from build123d import *

# Parameters (mm, degrees)
SKETCH2_W           = 101.6
SKETCH2_H           = 88.9
BOSS_EXTRUDE1_DEPTH = 3.175
SKETCH3_R           = 1.4605
CUT_EXTRUDE1_DEPTH  = 68.576054376
SKETCH5_W           = 3.175
SKETCH5_H           = 16.51
CUT_EXTRUDE2_DEPTH  = 68.576054376


with BuildPart() as part:
    # Sketch2 → Boss-Extrude1 (new body)
    with BuildSketch(Plane(origin=(0, 0, 0), x_dir=(1, 0, 0), z_dir=(0, 1, 0))):
        Rectangle(SKETCH2_W, SKETCH2_H)
    extrude(amount=BOSS_EXTRUDE1_DEPTH)

    # Sketch3 → Cut-Extrude1 (cut, through all)
    with BuildSketch(Plane(origin=(0, 3.175, 0), x_dir=(1, 0, 0), z_dir=(0, 1, 0))):
        with Locations(Location((-25.4, 0, 0), (0, 0, 270))):
            Circle(SKETCH3_R)
        with Locations(Location((25.4, 0, 0), (0, 0, 270))):
            Circle(SKETCH3_R)
    extrude(amount=-CUT_EXTRUDE1_DEPTH, mode=Mode.SUBTRACT)

    # Sketch5 → Cut-Extrude2 (cut, through all)
    with BuildSketch(Plane(origin=(0, 3.175, 0), x_dir=(1, 0, 0), z_dir=(0, 1, 0))):
        with Locations((-3.175, -1.713817512)):
            Rectangle(SKETCH5_W, SKETCH5_H)
        with Locations((3.175, -1.713817512)):
            Rectangle(SKETCH5_W, SKETCH5_H)
    extrude(amount=-CUT_EXTRUDE2_DEPTH, mode=Mode.SUBTRACT)


solid = part.part
Can you work these out from the model? Positions are in its coordinate system, mm. A direction names the side the tool comes from. Give positions to 0.01 mm unless a question says otherwise; leave off trailing zeros. Loops run counter-clockwise (first coordinate to the right, second up) from the corner with the lowest first, then second, coordinate; pieces in that order, holes last. Notation, with made-up numbers: (-16, -29.5) -> (42, -29.5) arc R29 ccw to (42, -2.5) -> close; hole circle Ø10 at (32.25, -5). An arc over 180 degrees is marked (long way). Return JSON: item names as keys, results as strings.
Q1. I want a section at B-B, the plane z = 0. List the corners of the cut face in (x, y) for me (1 decimal).
Checks:
{"outline": "(-50.8, 0) -> (-26.9, 0) -> (-26.9, 3.2) -> (-50.8, 3.2) -> close; (-23.9, 0) -> (-4.8, 0) -> (-4.8, 3.2) -> (-23.9, 3.2) -> close; (-1.6, 0) -> (1.6, 0) -> (1.6, 3.2) -> (-1.6, 3.2) -> close; (4.8, 0) -> (23.9, 0) -> (23.9, 3.2) -> (4.8, 3.2) -> close; (26.9, 0) -> (50.8, 0) -> (50.8, 3.2) -> (26.9, 3.2) -> close"}
Q2. We'd pull the mould along Z, two halves only. Please class faces 3 (the face through (3, 2, -6.541)), 4 (the face through (-1, 2, 44.45)), 5 (the face through (50.8, 2, 1)): released by +Z, released by -Z, zero draft, split by the parting line, or undercut.
Checks:
{"face 3": "undercut", "face 4": "released by +Z", "face 5": "zero draft"}
Q3. I need wall thicknesses on probe 1 along X at (y, z) = (1.7, 0); probe 2 along X at (y, z) = (1.4, 4.5); probe 3 along X at (y, z) = (1.45, 0.5). Which ranges of each line are inside material? Lowest first, please.
Checks:
{"probe 1": "x = -50.8 to -26.86, -23.94 to -4.76, -1.59 to 1.59, 4.76 to 23.94, 26.86 to 50.8", "probe 2": "x = -50.8 to -4.76, -1.59 to 1.59, 4.76 to 50.8", "probe 3": "x = -50.8 to -26.77, -24.03 to -4.76, -1.59 to 1.59, 4.76 to 24.03, 26.77 to 50.8"}
Q4. For pin 1 Ø1.8 at (x, z) = (25.4, 0) entering from -Y, with a flat end and sliding along its axis, tell me the tip position at first contact or that it passes through.
Checks:
{"pin 1": "passes through"}
Q5. On a 3-axis mill with a long thin cutter (end or side, diameter ignored), from which of +Z, -Z, +X, -X, +Y, -Y can I reach the whole of each face in a straight line? I mean faces 1 (the face through (-50.8, 2, 1)), 2 (the face through (-4.762, 2, 2)). Say none if no direction works.
Checks:
{"face 1": "+Z, -Z, -X, +Y, -Y", "face 2": "+Y, -Y"}
